Check sheet for the modelled part. Datum: model origin and axes. Units: mm. A direction names the side the tool comes from. Round coordinates to 2 decimals unless told otherwise and drop trailing zeros. Loops run counter-clockwise (first coordinate to the right, second up) from the corner with the lowest first, then second, coordinate; pieces in that order, holes last. Notation, with made-up numbers: (65, 35.5) -> (95, 35.5) arc R27 ccw to (95, 63.5) -> close; hole circle Ø9 at (85.25, 29.5). An arc over 180 degrees is marked (long way). Return JSON: item names as keys, results as strings.
from build123d import *

# Parameters (mm, degrees)
SKETCH1_W           = 33.5
SKETCH1_H           = 19.578427125
SKETCH1_R           = 1.5
SKETCH1_W_2         = 5.65685425
SKETCH1_H_2         = 5.65685425
BOSS_EXTRUDE1_DEPTH = 1
SKETCH1_3_W         = 5.65685425
SKETCH1_3_H         = 5.65685425
BOSS_EXTRUDE2_DEPTH = 49
SKETCH3_R           = 2.15
CUT_EXTRUDE1_DEPTH  = 2.25


with BuildPart() as part:
    # Sketch1 → Boss-Extrude1 (new body)
    # profile 1 of 2: a face of its own
    with BuildSketch(Plane(origin=(0, 0, 0), x_dir=(0, 0, -1), z_dir=(1, 0, 0))):
        with Locations((0, 6.960786437)):
            Rectangle(SKETCH1_W, SKETCH1_H)
        with Locations((8.485281374, 8.485281374)):
            Circle(SKETCH1_R, mode=Mode.SUBTRACT)
        with Locations((-8.485281374, 8.485281374)):
            Circle(SKETCH1_R, mode=Mode.SUBTRACT)
        with Locations((-14.75, 0)):
            Circle(SKETCH1_R, mode=Mode.SUBTRACT)
        with Locations((14.75, 0)):
            Circle(SKETCH1_R, mode=Mode.SUBTRACT)
        with Locations((0, 14.75)):
            Circle(SKETCH1_R, mode=Mode.SUBTRACT)
    # profile 2 of 2: a face of its own
    with BuildSketch(Plane(origin=(0, 0, 0), x_dir=(0, 0, -1), z_dir=(1, 0, 0))):
        Rectangle(SKETCH1_W_2, SKETCH1_H_2)
    extrude(amount=BOSS_EXTRUDE1_DEPTH)

    # Sketch1_3 → Boss-Extrude2 (add)
    with BuildSketch(Plane(origin=(0, 0, 0), x_dir=(0, 0, -1), z_dir=(1, 0, 0))):
        Rectangle(SKETCH1_3_W, SKETCH1_3_H)
    extrude(amount=BOSS_EXTRUDE2_DEPTH)

    # Sketch3 → Cut-Extrude1 (cut)
    with BuildSketch(Plane(origin=(49, 0, 0), x_dir=(0, 0, -1), z_dir=(1, 0, 0))):
        Circle(SKETCH3_R)
    extrude(amount=-CUT_EXTRUDE1_DEPTH, mode=Mode.SUBTRACT)


solid = part.part
Q1. Section check C-C (y = 0). Record the boundary of the cut face in (x, z).
Results list:
{"outline": "(0, -16.75) -> (1, -16.75) -> (1, -16.25) -> (0, -16.25) -> close; (0, -13.25) -> (1, -13.25) -> (1, -2.83) -> (49, -2.83) -> (49, -2.15) -> (46.75, -2.15) -> (46.75, 2.15) -> (49, 2.15) -> (49, 2.83) -> (1, 2.83) -> (1, 13.25) -> (0, 13.25) -> close; (0, 16.25) -> (1, 16.25) -> (1, 16.75) -> (0, 16.75) -> close"}
Q2. Tool access check on faces 5 (the flat face through (25, 0, -2.828)), 6 (the flat face through (46.75, 0, 0)), 7 (the flat face through (25, 0, 2.828)), 8 (the flat face through (25, 2.828, 0)). Record the directions out of +Z, -Z, +X, -X, +Y, -Y that give a thin tool (end or side, any length) a straight path to the whole face; none if there is none.
Results list:
{"face 5": "-Z, +X, +Y, -Y", "face 6": "+X", "face 7": "+Z, +X, +Y, -Y", "face 8": "+Z, -Z, +X, +Y"}
Q3. Draft check along Y on faces 1 (the flat face through (0.5, 16.75, 0.2)), 2 (the flat face through (0, 7, 0)), 3 (the cylindrical face through (47.89, 0.09, 2.15)), 4 (the flat face through (21, -2.828, 0)). Enter one of: released by +Y, released by -Y, zero draft, split by the parting line, or undercut.
Results list:
{"face 1": "released by +Y", "face 2": "zero draft", "face 3": "undercut", "face 4": "released by -Y"}
Q4. Go/stop test with flat-tipped pins: pin 1 (2.5 mm diameter, centred on y = 8.49, z = -8.49, fed in from +X); pin 2 (4.5 mm diameter, centred on x = 16, z = 0, fed in from +Y); pin 3 (1 mm diameter, centred on y = 2, z = 6, fed in from +X); pin 4 (6 mm diameter, centred on x = 16.5, y = 1, fed in from +Z). Record where each tip stops, or that it passes through.
Results list:
{"pin 1": "through", "pin 2": "y = 2.83", "pin 3": "x = 1", "pin 4": "z = 2.83"}
Q5. Section check B-B (y = 14.75). Record the boundary of the cut face in (x, z), then the cut area to 3 significant figures.
Results list:
{"outline": "(0, -16.75) -> (1, -16.75) -> (1, -1.5) -> (0, -1.5) -> close; (0, 1.5) -> (1, 1.5) -> (1, 16.75) -> (0, 16.75) -> close", "area": "30.5 mm^2"}
Q6. Material ranges on line 1 (Y direction, x = 0.4, z = 0); line 2 (X direction, y = 5.75, z = -9); line 3 (Y direction, x = 0.65, z = -14.75), recorded low to high.
Results list:
{"line 1": "-2.83 to 13.25, 16.25 to 16.75", "line 2": "0 to 1", "line 3": "-2.83 to -1.5, 1.5 to 16.75"}
Q7. Section check D-D (z = 0). Record the boundary of the cut face in (x, y).
Results list:
{"outline": "(0, -2.83) -> (49, -2.83) -> (49, -2.15) -> (46.75, -2.15) -> (46.75, 2.15) -> (49, 2.15) -> (49, 2.83) -> (1, 2.83) -> (1, 13.25) -> (0, 13.25) -> close; (0, 16.25) -> (1, 16.25) -> (1, 16.75) -> (0, 16.75) -> close"}
Q8. Section check A-A (z = 14.75). Record the boundary of the cut face in (x, y), then the cut area to 3 significant figures.
Results list:
{"outline": "(0, -2.83) -> (1, -2.83) -> (1, -1.5) -> (0, -1.5) -> close; (0, 1.5) -> (1, 1.5) -> (1, 16.75) -> (0, 16.75) -> close", "area": "16.6 mm^2"}
